from build123d import *

# Parameters (mm, degrees)
SKETCH2_R                = 33.8
CUT_EXTRUDE1_DEPTH       = 19.1
CUT_EXTRUDE2_START       = -33.8
CUT_EXTRUDE2_DEPTH       = 14.7
BOSS_EXTRUDE2_START      = -1.7
BOSS_EXTRUDE2_DEPTH      = 1.7
CUT_EXTRUDE3_REACH       = 42.172
SKETCH6_R                = 1.6
SKETCH19_R               = 9
CUT_EXTRUDE10_DEPTH      = 1.4
CUT_EXTRUDE11_REACH      = 42.429
CUT_EXTRUDE11_END_RADIUS = 33.8
SKETCH20_R               = 3.5
CUT_EXTRUDE9_REACH       = 44.024
CUT_EXTRUDE9_END_RADIUS  = 33.8
CUT_EXTRUDE7_REACH       = 44.024
CUT_EXTRUDE7_END_RADIUS  = 33.8
SKETCH10_R               = 1.6
CUT_EXTRUDE12_START      = -10.118299
SKETCH21_R               = 27.886018002
CUT_EXTRUDE12_DEPTH      = 10.118299
CUT_EXTRUDE13_REACH      = 41.529


# Read off the part's stored shape, not the designer's step: Revolve2
with BuildPart() as part:
    # Sketch1 → Revolve1 (revolve)
    with BuildSketch(Plane.XY, mode=Mode.PRIVATE) as revolve1_sk:
        with BuildLine():
            Line((0, -33.8), (0, 0))
            Line((0, 0), (33.8, 0))
            ThreePointArc((33.8, 0), (23.900209204, -23.900209204), (0, -33.8))
        make_face()
    revolve(revolve1_sk.sketch.rotate(Axis((0, -33.8, 0), (0, 1, 0)), 180), axis=Axis((0, -33.8, 0), (0, 1, 0)))

    # Sketch2 → Cut-Extrude1 (cut)
    with BuildSketch(Plane(origin=(0, 0, 0), x_dir=(1, 0, 0), z_dir=(0, 1, 0))):
        Circle(SKETCH2_R)
    extrude(amount=-CUT_EXTRUDE1_DEPTH, mode=Mode.SUBTRACT)

    # Sketch5 → Cut-Extrude2 (cut)
    with BuildSketch(Plane(origin=(0, 0, 0), x_dir=(1, 0, 0), z_dir=(0, 1, 0)).offset(CUT_EXTRUDE2_START)):
        with BuildLine():
            Line((-17.025732229, 6.571677263), (-23.544283672, 3.742739979))
            ThreePointArc((-23.544283672, 3.742739979), (-23.775794442, 3.633514413), (-24, 3.509985755))
            Line((-24, 3.509985755), (-24, -3.509985755))
            ThreePointArc((-24, -3.509985755), (-23.775794442, -3.633514413), (-23.544283672, -3.742739979))
            Line((-23.544283672, -3.742739979), (-17.025732229, -6.571677263))
            ThreePointArc((-17.025732229, -6.571677263), (0, -18.25), (17.025732229, -6.571677263))
            Line((17.025732229, -6.571677263), (23.544283672, -3.742739979))
            ThreePointArc((23.544283672, -3.742739979), (23.775794442, -3.633514413), (24, -3.509985755))
            Line((24, -3.509985755), (24, 3.509985755))
            ThreePointArc((24, 3.509985755), (23.775794442, 3.633514413), (23.544283672, 3.742739979))
            Line((23.544283672, 3.742739979), (17.025732229, 6.571677263))
            ThreePointArc((17.025732229, 6.571677263), (0, 18.25), (-17.025732229, 6.571677263))
        make_face()
    extrude(amount=CUT_EXTRUDE2_DEPTH, mode=Mode.SUBTRACT)

    # Sketch16 → Boss-Extrude2 (add)
    with BuildSketch(Plane(origin=(0, -19.1, 0), x_dir=(1, 0, 0), z_dir=(0, 1, 0)).offset(BOSS_EXTRUDE2_START)):
        with BuildLine():
            Line((17.025732229, 6.571677263), (23.544283672, 3.742739979))
            ThreePointArc((23.544283672, 3.742739979), (23.775794442, 3.633514413), (24, 3.509985755))
            Line((24, 3.509985755), (24, -3.509985755))
            ThreePointArc((24, -3.509985755), (23.775794442, -3.633514413), (23.544283672, -3.742739979))
            Line((23.544283672, -3.742739979), (17.025732229, -6.571677263))
            ThreePointArc((17.025732229, -6.571677263), (18.25, 0), (17.025732229, 6.571677263))
        make_face()
        with BuildLine():
            Line((-23.544283672, -3.742739979), (-17.025732229, -6.571677263))
            ThreePointArc((-17.025732229, -6.571677263), (-18.25, 0), (-17.025732229, 6.571677263))
            Line((-17.025732229, 6.571677263), (-23.544283672, 3.742739979))
            ThreePointArc((-23.544283672, 3.742739979), (-23.775794442, 3.633514413), (-24, 3.509985755))
            Line((-24, 3.509985755), (-24, -3.509985755))
            ThreePointArc((-24, -3.509985755), (-23.775794442, -3.633514413), (-23.544283672, -3.742739979))
        make_face()
    extrude(amount=BOSS_EXTRUDE2_DEPTH)

    # Sketch6 → Cut-Extrude3 (cut, up to next)
    with BuildSketch(Plane(origin=(0, -20.8, 0), x_dir=(1, 0, 0), z_dir=(0, 1, 0)), mode=Mode.PRIVATE) as cut_extrude3_sk1:
        with Locations(Location((-21.92, 0, 0), (0, 0, 270))):
            Circle(SKETCH6_R)
    cut_extrude3_tool1 = extrude(cut_extrude3_sk1.sketch, amount=CUT_EXTRUDE3_REACH, mode=Mode.PRIVATE) & part.part
    # Sketch6 → Cut-Extrude3 (cut, up to next)
    with BuildSketch(Plane(origin=(0, -20.8, 0), x_dir=(1, 0, 0), z_dir=(0, 1, 0)), mode=Mode.PRIVATE) as cut_extrude3_sk2:
        with Locations(Location((21.92, 0, 0), (0, 0, 270))):
            Circle(SKETCH6_R)
    cut_extrude3_tool2 = extrude(cut_extrude3_sk2.sketch, amount=CUT_EXTRUDE3_REACH, mode=Mode.PRIVATE) & part.part
    add(cut_extrude3_tool1.solids().sort_by_distance((-21.92, -20.8, 0))[0], mode=Mode.SUBTRACT)
    add(cut_extrude3_tool2.solids().sort_by_distance((21.92, -20.8, 0))[0], mode=Mode.SUBTRACT)

    # Revolve2 outline → Revolve2 (revolve)
    with BuildSketch(Plane.XY):
        with BuildLine():
            Line((0, -23.5), (0, -33.8))
            ThreePointArc((0, -33.8), (13.168073663, -31.129436808), (24.255308697, -23.53975361))
            Line((24.255308697, -23.53975361), (24.255308697, -23.5))
            Line((24.255308697, -23.5), (0, -23.5))
        make_face()
    revolve(axis=Axis((0, 0, 0), (0, 1, 0)))

    # Sketch19 → Cut-Extrude10 (cut)
    with BuildSketch(Plane(origin=(0, -23.5, 0), x_dir=(1, 0, 0), z_dir=(0, 1, 0))):
        with Locations(Location((0, 0, 0), (0, 0, 180))):
            Circle(SKETCH19_R)
    extrude(amount=-CUT_EXTRUDE10_DEPTH, mode=Mode.SUBTRACT)

    # Cut-Extrude11: up to this sphere (the profile starts inside it)
    cut_extrude11_end = Location((0, 0, 0)) * Sphere(CUT_EXTRUDE11_END_RADIUS, mode=Mode.PRIVATE)
    # Sketch20 → Cut-Extrude11 (cut, up to the surface)
    with BuildSketch(Plane(origin=(0, -24.9, 0), x_dir=(1, 0, 0), z_dir=(0, 1, 0)), mode=Mode.PRIVATE) as cut_extrude11_sk1:
        with Locations(Location((0, 0, 0), (0, 0, 180))):
            Circle(SKETCH20_R)
    cut_extrude11_tool1 = extrude(cut_extrude11_sk1.sketch, amount=-CUT_EXTRUDE11_REACH, mode=Mode.PRIVATE) & cut_extrude11_end
    add(cut_extrude11_tool1.solids().sort_by_distance((0, -24.9, 0))[0], mode=Mode.SUBTRACT)

    # Cut-Extrude9: up to this sphere (the profile starts inside it)
    cut_extrude9_end = Location((0, 0, 0)) * Sphere(CUT_EXTRUDE9_END_RADIUS, mode=Mode.PRIVATE)
    # Sketch13 → Cut-Extrude9 (cut, up to the surface)
    with BuildSketch(Plane(origin=(0, -19.1, 0), x_dir=(1, 0, 0), z_dir=(0, 1, 0)), mode=Mode.PRIVATE) as cut_extrude9_sk1:
        Polygon((10.556374993, -19.224020053), (13.210464636, -21.224020053), (17.724077309, -15.234253728), (16.925441799, -14.632438705), (18.730886869, -12.236532175), (19.529522379, -12.838347198), (24.043135053, -6.848580873), (21.389045409, -4.848580873), align=None)
    cut_extrude9_tool1 = extrude(cut_extrude9_sk1.sketch, amount=-CUT_EXTRUDE9_REACH, mode=Mode.PRIVATE) & cut_extrude9_end
    add(cut_extrude9_tool1.solids().sort_by_distance((17.250772, -19.1, 12.999389))[0], mode=Mode.SUBTRACT)

    # Cut-Extrude7: up to this sphere (the profile starts inside it)
    cut_extrude7_end = Location((0, 0, 0)) * Sphere(CUT_EXTRUDE7_END_RADIUS, mode=Mode.PRIVATE)
    # Sketch10 → Cut-Extrude7 (cut, up to the surface)
    with BuildSketch(Plane(origin=(0, -19.1, 0), x_dir=(1, 0, 0), z_dir=(0, 1, 0)), mode=Mode.PRIVATE) as cut_extrude7_sk1:
        with Locations(Location((-18.186533479, -10.5, 0), (0, 0, 270))):
            Circle(SKETCH10_R)
    cut_extrude7_tool1 = extrude(cut_extrude7_sk1.sketch, amount=-CUT_EXTRUDE7_REACH, mode=Mode.PRIVATE) & cut_extrude7_end
    add(cut_extrude7_tool1.solids().sort_by_distance((-18.186533, -19.1, 10.5))[0], mode=Mode.SUBTRACT)
    # Sketch10 → Cut-Extrude7 (cut, up to the surface)
    with BuildSketch(Plane(origin=(0, -19.1, 0), x_dir=(1, 0, 0), z_dir=(0, 1, 0)), mode=Mode.PRIVATE) as cut_extrude7_sk2:
        with Locations(Location((18.186533479, 10.5, 0), (0, 0, 270))):
            Circle(SKETCH10_R)
    cut_extrude7_tool2 = extrude(cut_extrude7_sk2.sketch, amount=-CUT_EXTRUDE7_REACH, mode=Mode.PRIVATE) & cut_extrude7_end
    add(cut_extrude7_tool2.solids().sort_by_distance((18.186533, -19.1, -10.5))[0], mode=Mode.SUBTRACT)

    # Sketch21 → Cut-Extrude12 (cut)
    with BuildSketch(Plane(origin=(0, -23.5, 0), x_dir=(1, 0, 0), z_dir=(0, 1, 0)).offset(CUT_EXTRUDE12_START)):
        Circle(SKETCH21_R)
    extrude(amount=CUT_EXTRUDE12_DEPTH, mode=Mode.SUBTRACT)

    # Sketch23 → Cut-Extrude13 (cut, up to next)
    with BuildSketch(Plane.XZ.offset(20.8), mode=Mode.PRIVATE) as cut_extrude13_sk1:
        Polygon((24, 3.509985755), (24, -3.509985755), (29.923076923, 0), align=None)
    cut_extrude13_tool1 = extrude(cut_extrude13_sk1.sketch, amount=CUT_EXTRUDE13_REACH, mode=Mode.PRIVATE) & part.part
    # Sketch23 → Cut-Extrude13 (cut, up to next)
    with BuildSketch(Plane.XZ.offset(20.8), mode=Mode.PRIVATE) as cut_extrude13_sk2:
        Polygon((-24, 3.509985755), (-24, -3.509985755), (-29.923076923, 0), align=None)
    cut_extrude13_tool2 = extrude(cut_extrude13_sk2.sketch, amount=CUT_EXTRUDE13_REACH, mode=Mode.PRIVATE) & part.part
    add(cut_extrude13_tool1.solids().sort_by_distance((25.974359, -20.8, 0))[0], mode=Mode.SUBTRACT)
    add(cut_extrude13_tool2.solids().sort_by_distance((-25.974359, -20.8, 0))[0], mode=Mode.SUBTRACT)


solid = part.part
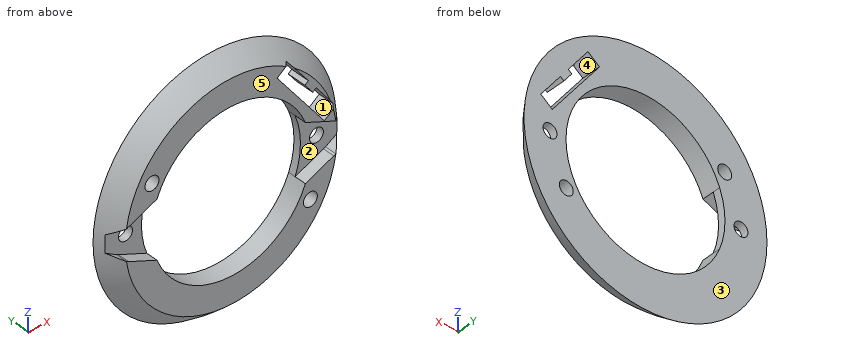
Work out the finished part from the listing and answer in its coordinate system (mm). Face numbers are marked on the shaded views. A direction names the side the tool comes from. Round coordinates to 2 decimals unless told otherwise and drop trailing zeros. Write each loop counter-clockwise with the first axis right and the second up, starting at its lowest first coordinate (ties: lowest second). Pieces come first, ordered by that corner, then holes.
1) A cutting plane is placed at A-A (y = -21.7). Give the vertices of the cut face in (x, z), plus the area to 3 significant figures.
2) The mould has two halves that part along Z. Classify the marked faces 4 and 5: pulls with the +Z half, pulls with the -Z half, needs draft (parallel to the pull), parting line crosses it, or undercut.
3) Straight lines are drawn through the part: line 1 (X direction, y = -20.3, z = 0); line 2 (X direction, y = -22.25, z = 8); line 3 (X direction, y = -20.1, z = -10.5). For each, find the intervals that lie inside material, in ascending order.
4) A cutting plane is placed at C-C (x = -21.92). Give the vertices of the cut face in (y, z), plus the area to 3 significant figures.
5) A tool of negligible diameter and unlimited length cuts with its end or side. For the marked faces 1, 2 and 3, from which of +Z, -Z, +X, -X, +Y, -Y can it reach the whole face along a straight path? Write none if from no direction.
6) A cutting plane is placed at B-B (z = 0). Give the vertices of the cut face in (x, y), plus the area to 3 significant figures.
7) Given pin 1 Ø2 at (x, y) = (18, -21.5) entering from +Z; pin 2 Ø1 at (x, z) = (-20, 2) entering from -Y; pin 3 Ø1.5 at (y, z) = (-21, -10) entering from -X, each flat-ended and moving along its own axis, determine where each tip first touches the part or whether it passes through.
8) A cutting plane is placed at D-D (z = -10.5). Give the vertices of the cut face in (x, y).
Completed:
1. outline: (-25.8, -2.44) arc R25.91 ccw to (25.8, -2.44) - (24, -3.51) arc R4.08 cw to (23.54, -3.74) - (17.03, -6.57) arc R18.25 cw to (-17.03, -6.57) - (-23.54, -3.74) arc R4.08 cw to (-24, -3.51) - close; (-25.8, 2.44) - (-24, 3.51) arc R4.08 cw to (-23.54, 3.74) - (-17.03, 6.57) arc R18.25 cw to (17.03, 6.57) - (23.54, 3.74) arc R4.08 cw to (24, 3.51) - (25.8, 2.44) arc R25.91 ccw to start; hole circle Ø3.2 at (-18.19, 10.5); hole (10.56, 19.22) - (21.39, 4.85) - (24.04, 6.85) - (19.53, 12.84) - (18.73, 12.24) - (16.93, 14.63) - (17.72, 15.23) - (13.21, 21.22) - close; hole circle Ø3.2 at (18.19, -10.5)
1. area: 849 mm2
2. face 4: undercut
2. face 5: needs draft
3. line 1: x = -27.02 to -23.52, -20.32 to -18.25, 18.25 to 20.32, 23.52 to 27.02
3. line 2: x = -24.15 to -16.4, 16.4 to 19.01, 23.18 to 24.15
3. line 3: x = -25.06 to -14.93, 14.93 to 16.59, 19.79 to 25.06
4. outline: (-23.5, -10.47) arc R25.73 ccw to (-19.1, -17.24) - (-19.1, -1.6) - (-20.8, -1.6) - (-20.8, -4.45) - (-23.5, -4.45) - close; (-23.5, 4.45) - (-20.8, 4.45) - (-20.8, 1.6) - (-19.1, 1.6) - (-19.1, 17.24) arc R25.73 ccw to (-23.5, 10.47) - close
4. area: 95.9 mm2
5. face 1: +Y, -Y
5. face 2: -Y
5. face 3: +Z, -Z, +X, -X, +Y
6. outline: (-27.89, -19.1) arc R33.8 ccw to (-26.64, -20.8) - (-23.52, -20.8) - (-23.52, -19.1) - close; (-20.32, -20.8) - (-18.25, -20.8) - (-18.25, -19.1) - (-20.32, -19.1) - close; (18.25, -20.8) - (20.32, -20.8) - (20.32, -19.1) - (18.25, -19.1) - close; (23.52, -20.8) - (26.64, -20.8) arc R33.8 ccw to (27.89, -19.1) - (23.52, -19.1) - close
6. area: 19.8 mm2
7. pin 1: stops at z = 20.28
7. pin 2: stops at y = -20.8
7. pin 3: stops at x = -25.21
8. outline: (-25.83, -19.1) arc R32.13 ccw to (-21.91, -23.5) - (-14.93, -23.5) - (-14.93, -19.1) - close; (14.93, -23.5) - (16.59, -23.5) - (16.59, -19.1) - (14.93, -19.1) - close; (19.79, -23.5) - (21.91, -23.5) arc R32.13 ccw to (25.83, -19.1) - (19.79, -19.1) - close
